Geometry: see drawing. Coordinates: mm, zero at the bounding-box minimum. A direction names the side the tool comes from. Give positions to 0.01 mm unless a question says otherwise; leave off trailing zeros. Write each loop counter-clockwise with the first axis right and the second up, starting at its lowest first coordinate (ties: lowest second). Pieces come first, ordered by that corner, then holes. Notation, with made-up numbers: (-6, 36.5) -> (40, 36.5) arc R7 ccw to (40, 40.5) -> close; hole circle Ø9 at (45.5, -5.75). An arc over 180 degrees is marked (long way). Answer as a JSON object with one key per item and string values. Group by question number.
Item 1: Access query for the marked faces 1, 2 and 3. Directions: +Z, -Z, +X, -X, +Y, -Y. A direction counts if a zero-diameter tool reaches every point of the face in a straight line with its end or side. Return the directions, or none.
Item 2: Section query D-D on x = 9.75. Return the cut outline in (y, z).
Item 3: Section query C-C on y = 5. Return the cut outline in (x, z) (1 decimal).
Item 4: Ray query, probe 1 along Z at (x, y) = (9.75, 12.5); probe 2 along Z at (x, y) = (7, 20); probe 3 along Y at (x, z) = (18, 16.5). Return the intervals inside material, ascending. Write a range as from..to.
Item 5: Section query B-B on x = 1.5. Return the cut outline in (y, z).
Item 6: First-contact query: pin 1 Ø2.5 at (x, y) = (4.65, 5.5) entering from +Z; pin 2 Ø10 at (x, z) = (7, 9) entering from +Y; pin 3 Ø3 at (x, z) = (14, 11) entering from -Y; pin 4 Ø4 at (x, y) = (14.85, 5.5) entering from -Z. Flat tips, straight axial feed; report the tip coordinate or a pass-through.
Item 7: Section query A-A on z = 9.75. Return the cut outline in (x, y), plus the area to 3 significant figures.
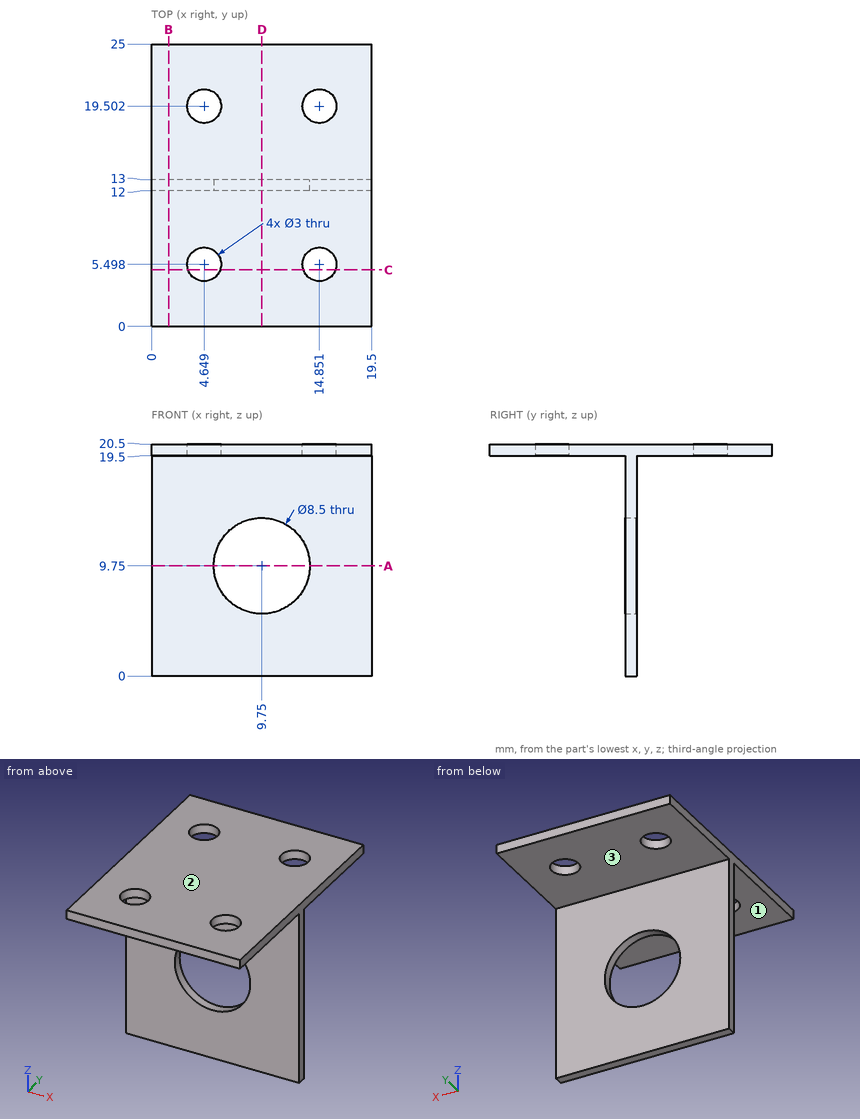
Worked answers:
{
 "1": {"face 1": "-Z, +X, -X, -Y", "face 2": "+Z, +X, -X, +Y, -Y", "face 3": "-Z, +X, -X, +Y"},
 "2": {"outline": "(0, 19.5) -> (12, 19.5) -> (12, 14) -> (13, 14) -> (13, 19.5) -> (25, 19.5) -> (25, 20.5) -> (0, 20.5) -> close; (12, 0) -> (13, 0) -> (13, 5.5) -> (12, 5.5) -> close"},
 "3": {"outline": "(0, 19.5) -> (3.2, 19.5) -> (3.2, 20.5) -> (0, 20.5) -> close; (6.1, 19.5) -> (13.4, 19.5) -> (13.4, 20.5) -> (6.1, 20.5) -> close; (16.3, 19.5) -> (19.5, 19.5) -> (19.5, 20.5) -> (16.3, 20.5) -> close"},
 "4": {"probe 1": "0..5.5, 14..20.5", "probe 2": "19.5..20.5", "probe 3": "12..13"},
 "5": {"outline": "(0, 19.5) -> (12, 19.5) -> (12, 0) -> (13, 0) -> (13, 19.5) -> (25, 19.5) -> (25, 20.5) -> (0, 20.5) -> close"},
 "6": {"pin 1": "through", "pin 2": "y = 13", "pin 3": "y = 12", "pin 4": "z = 19.5"},
 "7": {"outline": "(0, 12) -> (5.5, 12) -> (5.5, 13) -> (0, 13) -> close; (14, 12) -> (19.5, 12) -> (19.5, 13) -> (14, 13) -> close", "area": "11.0 mm^2"}
}
